```python
from build123d import *

# Parameters (mm, degrees)
SKETCH_1_W                  = 55
SKETCH_1_H                  = 46
EXTRUDE_1_DEPTH             = 46
SKETCH_2_R                  = 19
EXTRUDE_2_DEPTH             = 2
FILLET_1_R                  = 0.3
HOLE_WIZARD_11_0_11_1_D     = 11
HOLE_WIZARD_11_0_11_1_DEPTH = 2
SKETCH_5_R                  = 3.175
EXTRUDE_3_DEPTH             = 21
CUT_EXTRUDE_START           = -18
CUT_EXTRUDE_1_DEPTH         = 18
HOLE_WIZARD_8_0_8_1_DEPTH   = 55
HOLE_WIZARD_5_2_5_2_2_D     = 5.2
HOLE_WIZARD_5_2_5_2_2_DEPTH = 55
HOLE_WIZARD_2_0_2_1_D       = 2
HOLE_WIZARD_2_0_2_1_DEPTH   = 10
CHAMFER_1_SIZE              = 0.5
CHAMFER_2_SIZE              = 0.1
SKETCH_15_R                 = 21
EXTRUDE_4_DEPTH             = 30
SKETCH_16_W                 = 43
SKETCH_16_H                 = 43
EXTRUDE_5_DEPTH             = 7
CHAMFER_3_SIZE              = 2


# Read off the part's stored shape, not the designer's step: Ø8.0 (8) 直径孔1
with BuildPart() as part:
    # 草图1 → 凸台-拉伸1 (new body)
    with BuildSketch(Plane(origin=(28, 0, 0), x_dir=(0, 0, -1), z_dir=(1, 0, 0))):
        with Locations((-27.5, 0)):
            Rectangle(SKETCH_1_W, SKETCH_1_H)
    extrude(amount=-EXTRUDE_1_DEPTH)

    # 草图2 → 凸台-拉伸2 (add)
    with BuildSketch(Plane.XY.offset(55)):
        with Locations((4.421826919, 0)):
            Circle(SKETCH_2_R)
    extrude(amount=EXTRUDE_2_DEPTH)

    # 圆角1
    fillet_1_edges = [part.edges().sort_by_distance(p)[0] for p in [
        (-14.578173081, 0, 55),
    ]]
    fillet(fillet_1_edges, radius=FILLET_1_R)

    # Ø11.0 (11) 直径孔1
    with Locations(Plane.XY.offset(57)):
        with Locations((0, 0)):
            Hole(HOLE_WIZARD_11_0_11_1_D / 2, depth=HOLE_WIZARD_11_0_11_1_DEPTH)

    # 草图5 → 凸台-拉伸3 (add)
    with BuildSketch(Plane.XY.offset(55)):
        with Locations(Location((0, 0, 0), (0, 0, 180))):
            Circle(SKETCH_5_R)
    extrude(amount=EXTRUDE_3_DEPTH)

    # 草图6 → 切除-拉伸1 (cut)
    with BuildSketch(Plane.XY.offset(76).offset(CUT_EXTRUDE_START)):
        with BuildLine():
            Line((-2.107130751, 2.375), (2.107130751, 2.375))
            ThreePointArc((2.107130751, 2.375), (0, 3.175), (-2.107130751, 2.375))
        make_face()
    extrude(amount=CUT_EXTRUDE_1_DEPTH, mode=Mode.SUBTRACT)

    # Ø8.0 (8) 直径孔1 outline → Ø8.0 (8) 直径孔1 (cut)
    with BuildSketch(Plane.XY):
        with BuildLine():
            ThreePointArc((-12.354248689, -23), (-12.171572875, -17.171572875), (-18, -17.354248689))
            Line((-18, -17.354248689), (-18, -23))
            Line((-18, -23), (-12.354248689, -23))
        make_face()
        with BuildLine():
            Line((-18, 23), (-18, 17.354248689))
            ThreePointArc((-18, 17.354248689), (-12.171572875, 17.171572875), (-12.354248689, 23))
            Line((-12.354248689, 23), (-18, 23))
        make_face()
        with BuildLine():
            ThreePointArc((28, -17.354248689), (22.171572875, -17.171572875), (22.354248689, -23))
            Line((22.354248689, -23), (28, -23))
            Line((28, -23), (28, -17.354248689))
        make_face()
        with BuildLine():
            Line((28, 23), (22.354248689, 23))
            ThreePointArc((22.354248689, 23), (22.171572875, 17.171572875), (28, 17.354248689))
            Line((28, 17.354248689), (28, 23))
        make_face()
    extrude(amount=HOLE_WIZARD_8_0_8_1_DEPTH, mode=Mode.SUBTRACT)

    # Ø5.2 (5.2) 直径孔2
    with Locations(Plane.XY.offset(55)):
        with Locations((23.5, 23.5), (23.5, -23.5), (-23.5, 23.5)):
            Hole(HOLE_WIZARD_5_2_5_2_2_D / 2, depth=HOLE_WIZARD_5_2_5_2_2_DEPTH)

    # Ø2.0 (2) 直径孔1
    with Locations(Plane.XY.offset(76)):
        with Locations((0, 0)):
            Hole(HOLE_WIZARD_2_0_2_1_D / 2, depth=HOLE_WIZARD_2_0_2_1_DEPTH)

    # 倒角1
    chamfer_1_edges = [part.edges().sort_by_distance(p)[0] for p in [
        (1.302014759, -2.895752504, 76),
        (0, 2.375, 76),
    ]]
    chamfer(chamfer_1_edges, length=CHAMFER_1_SIZE)

    # 倒角2
    chamfer_2_edges = [part.edges().sort_by_distance(p)[0] for p in [
        (1, 0, 76),
    ]]
    chamfer(chamfer_2_edges, length=CHAMFER_2_SIZE)

    # 草图15 → 凸台-拉伸4 (add)
    with BuildSketch(Plane.XY.offset(57)):
        with Locations((5.5, 0)):
            Circle(SKETCH_15_R)
    extrude(amount=EXTRUDE_4_DEPTH)

    # 草图16 → 凸台-拉伸5 (add)
    with BuildSketch(Plane.XY.offset(87)):
        with Locations((5.5, 0)):
            Rectangle(SKETCH_16_W, SKETCH_16_H)
    extrude(amount=EXTRUDE_5_DEPTH)

    # 倒角3
    chamfer_3_edges = [part.edges().sort_by_distance(p)[0] for p in [
        (27, -21.5, 90.5),
        (27, 21.5, 90.5),
        (-16, 21.5, 90.5),
        (-16, -21.5, 90.5),
    ]]
    chamfer(chamfer_3_edges, length=CHAMFER_3_SIZE)


solid = part.part
```
Verification items for the finished model (mm, model axes). A direction names the side the tool comes from. Coordinates: 2 decimals unless noted, no trailing zeros. Loops run counter-clockwise (first coordinate to the right, second up) from the corner with the lowest first, then second, coordinate; pieces in that order, holes last. Notation, with made-up numbers: (36, 31) -> (79, 31) arc R13 ccw to (79, 49) -> close; hole circle Ø3 at (-9, -22.75). An arc over 180 degrees is marked (long way). Answer in a Markdown table with one row per item. Add a question column.
1. Section check B-B, the plane z = 43.5. Enter the section's corners in (x, y).
2. Section check A-A, the plane y = 0. Enter the section's corners in (x, z) (3 decimals).
3. Draft check along Z on faces 6 (the face through (1.19, -5.37, 55.99)), 7 (the face through (5, 0, 0)), 8 (the face through (5, -21.5, 90)), 9 (the face through (5, 0, 94)). Enter one of: +Z half, -Z half, draft (parallel to the pull), parting line (faces both ways), or undercut.
4. Section check C-C, the plane z = 64. Enter the section's corners in (x, y).
5. Access from +Z, -Z, +X, -X, +Y, -Y to the whole of each face (thin tool, end or side, straight path). Record for faces 1 (the face through (-18, 0, 28)), 2 (the face through (27, 0, 90)), 3 (the face through (22.656, 16.759, 27.115)), 4 (the face through (23, -6, 57)), 5 (the face through (26, -20.5, 90.5)).
6. Material ranges on probe 1 along Z at (x, y) = (-15, 13); probe 2 along Z at (x, y) = (23, 6); probe 3 along Y at (x, z) = (0, 56.1) (3 decimals), recorded low to high. Write a range as [from, to].
7. Depth check by flat-ended pin: P1, Ø6, axis at x = 9.5, z = 78.5, coming from the +Y side; P2, Ø7.5, axis at y = 6.5, z = 90.5, coming from the -X side; P3, Ø8, axis at y = 10, z = 73, coming from the -X side; P4, Ø3, axis at x = 23, y = 0, coming from the -Z side. Enter the tip coordinate at first touch or a pass-through.
Derived:
| question | item | result |
|---|---|---|
| 1 | outline | (-18, -17.35) arc R4 cw (long way) to (-12.35, -23) -> (20.95, -23) arc R2.6 cw to (21.47, -21.88) arc R4 cw to (28, -17.35) -> (28, 17.35) arc R4 cw to (21.47, 21.88) arc R2.6 cw to (20.95, 23) -> (-12.35, 23) arc R4 cw (long way) to (-18, 17.35) -> close |
| 2 | outline | (-18, 0) -> (28, 0) -> (28, 55) -> (23.722, 55) arc R0.3 cw to (23.422, 55.3) -> (23.422, 57) -> (26.5, 57) -> (26.5, 87) -> (27, 87) -> (27, 94) -> (-16, 94) -> (-16, 87) -> (-15.5, 87) -> (-15.5, 57) -> (-14.578, 57) -> (-14.578, 55.3) arc R0.3 cw to (-14.878, 55) -> (-18, 55) -> close; hole (-5.5, 55) -> (-3.175, 55) -> (-3.175, 57) -> (-5.5, 57) -> close; hole (3.175, 55) -> (5.5, 55) -> (5.5, 57) -> (3.175, 57) -> close |
| 3 | face 6 | undercut |
| 3 | face 7 | -Z half |
| 3 | face 8 | draft |
| 3 | face 9 | +Z half |
| 4 | outline | circle Ø42 at (5.5, 0) |
| 5 | face 1 | +Z, -Z, -X, +Y, -Y |
| 5 | face 2 | +Z, +X, +Y, -Y |
| 5 | face 3 | -Z |
| 5 | face 4 | none |
| 5 | face 5 | +Z, -Z, +X, -Y |
| 6 | probe 1 | z = [0, 55], [87, 94] |
| 6 | probe 2 | z = [0, 55], [57, 94] |
| 6 | probe 3 | y = [-18.478, -5.5], [-3.175, 3.175], [5.5, 18.478] |
| 7 | P1 | stops at y = 20.98 |
| 7 | P2 | stops at x = -16 |
| 7 | P3 | stops at x = -14.62 |
| 7 | P4 | stops at z = 0 |
